Verification items for the finished model (mm, model axes). A direction names the side the tool comes from. Give positions to 0.01 mm unless a question says otherwise; leave off trailing zeros. Write each loop counter-clockwise with the first axis right and the second up, starting at its lowest first coordinate (ties: lowest second). Pieces come first, ordered by that corner, then holes.
Autodesk Inventor part; units mm, degrees
ref_plane "YZ Plane" through (0, 0, 0) normal (1, 0, 0) x (0, 1, 0)
ref_plane "XZ Plane" through (0, 0, 0) normal (0, 1, 0) x (-1, 0, 0)
ref_plane "XY Plane" through (0, 0, 0) normal (0, 0, 1) x (1, 0, 0)
sketch "Skizze1" plane through (0, 0, 0) normal (0, 0, 1) x (1, 0, 0)
  line L0 (-20.9977, -1.3) -> (5.0023, -1.3)
  line L1 (-22.2477, 0) -> (6.2523, 0)
  line L2 (-22.2477, 0) -> (-22.2477, -2.7)
  line L3 (-22.2477, -2.7) -> (-20.9977, -2.7)
  line L4 (-20.9977, -2.7) -> (-20.9977, -1.3)
  line L5 (5.0023, -1.3) -> (5.0023, -2.7)
  line L6 (5.0023, -2.7) -> (6.2523, -2.7)
  line L7 (6.2523, -2.7) -> (6.2523, 0)
  point P0 (0, 0)
  dimension "d0" = 26
  dimension "d1" = 28.5
  dimension "d2" = 1.25
  dimension "d33" = 1.3
  dimension "d37" = 2.7
  dimension "d38" = 2.7
  dimension "d39" = 0
extrude "Extrusion1" add sketch "Skizze1" along normal blind 25.5
sketch "Skizze2" plane through (0, 0, 0) normal (0, 0, -1) x (-1, 0, 0)
  line L0 (20.9977, -1.3) -> (-5.0023, -1.3)
  line L1 (20.9977, -2.7) -> (20.9977, -1.3)
  line L2 (-5.0023, -1.3) -> (-5.0023, -2.7)
  line L3 (0.9977, -1.3) -> (2.2477, -1.3)
  line L4 (2.2477, -1.3) -> (2.2477, -5.5195)
  line L5 (2.2477, -5.5195) -> (0.9977, -5.5195)
  line L6 (0.9977, -5.5195) -> (0.9977, -1.3)
  line L7 (13.7477, -1.3) -> (14.9977, -1.3)
  line L8 (14.9977, -1.3) -> (14.9977, -5.5195)
  line L9 (14.9977, -5.5195) -> (13.7477, -5.5195)
  line L10 (13.7477, -5.5195) -> (13.7477, -1.3)
  point P0 (0, 0)
  dimension "d5" = 11.5
  dimension "d6" = 1.25
  dimension "d7" = 1.25
  dimension "d8" = 6
  dimension "d9" = 6
extrude "Extrusion2" add sketch "Skizze2" against normal blind 16.35
sketch "Skizze3" plane through (0, 0, 0) normal (0, 0, -1) x (-1, 0, 0)
  line L0 (0.9977, -5.5195) -> (2.2477, -5.5195)
  line L1 (2.2477, -5.5195) -> (2.2477, -17.7695)
  line L2 (2.2477, -17.7695) -> (0.9977, -17.7695)
  line L3 (0.9977, -17.7695) -> (0.9977, -5.5195)
  line L4 (13.7477, -5.5195) -> (14.9977, -5.5195)
  line L5 (14.9977, -5.5195) -> (14.9977, -17.7695)
  line L6 (14.9977, -17.7695) -> (13.7477, -17.7695)
  line L7 (13.7477, -17.7695) -> (13.7477, -5.5195)
  point P0 (0, 0)
  dimension "d12" = 12.25
  dimension "d15" = 12.25
extrude "Extrusion3" add sketch "Skizze3" against normal blind 5
sketch "Skizze4" plane through (0, 0, 0) normal (0, 0, -1) x (-1, 0, 0)
  line L0 (0.9977, -17.7695) -> (2.2477, -17.7695)
  line L1 (2.2477, -17.7695) -> (2.2477, -24.0195)
  line L2 (2.2477, -24.0195) -> (0.9977, -24.0195)
  line L3 (0.9977, -24.0195) -> (0.9977, -17.7695)
  line L4 (13.7477, -17.7695) -> (14.9977, -17.7695)
  line L5 (14.9977, -17.7695) -> (14.9977, -24.0195)
  line L6 (14.9977, -24.0195) -> (13.7477, -24.0195)
  line L7 (13.7477, -24.0195) -> (13.7477, -17.7695)
  point P0 (0, 0)
  dimension "d16" = 6.25
  dimension "d17" = 6.25
extrude "Extrusion4" add sketch "Skizze4" against normal blind 16.35
sketch "Skizze5" plane through (-14.9977, -24.0195, 0) normal (0, -1, 0) x (1, 0, 0)
  line L0 (-7.25, 0) -> (-7.25, 25.5)
  line L1 (21.25, 0) -> (21.25, 25.5)
  line L2 (-7.25, 25.5) -> (-7.25, 0)
  line L3 (21.25, 0) -> (-7.25, 0)
  line L4 (21.25, 0) -> (21.25, 25.5)
  line L5 (21.25, 25.5) -> (18.8, 25.5)
  line L6 (18.8, 25.5) -> (18.8, 5.0223)
  line L7 (18.8, 5.0223) -> (15, 5.0223)
  line L8 (15, 5.0223) -> (15, 25.5)
  line L9 (15, 25.5) -> (6.75, 25.5)
  line L10 (6.75, 25.5) -> (6.75, 5.25)
  line L11 (6.75, 5.25) -> (-3.25, 5.25)
  line L12 (-3.25, 5.25) -> (-3.25, 25.5)
  line L13 (-3.25, 25.5) -> (-7.25, 25.5)
  point P0 (14.9977, 0)
  dimension "d20" = 5.25
  dimension "d21" = 8.25
  dimension "d22" = 3.8
  dimension "d23" = 10
  dimension "d24" = 4
  dimension "d25" = 2.45
extrude "Extrusion5" add sketch "Skizze5" against normal blind 1.3
sketch "Skizze6" plane through (-14.9977, -22.7195, 0) normal (0, 1, 0) x (1, 0, 0)
  line L0 (-3.25, -25.5) -> (-7.25, -25.5)
  line L1 (14, 0) -> (21.25, 0)
  line L2 (21.25, -25.5) -> (21.25, 0)
  line L3 (-7.25, 0) -> (-6, 0)
  line L4 (-6, 0) -> (-6, -25.5)
  line L5 (-6, -25.5) -> (-7.25, -25.5)
  line L6 (-7.25, -25.5) -> (-7.25, 0)
  line L7 (21.25, 0) -> (20, 0)
  line L8 (20, 0) -> (20, -25.5)
  line L9 (20, -25.5) -> (21.25, -25.5)
  line L10 (21.25, -25.5) -> (21.25, 0)
  point P0 (14.9977, 0)
  point P1 (18.8, -25.5)
  dimension "d28" = 1.25
  dimension "d30" = 1.25
extrude "Extrusion6" add sketch "Skizze6" along normal blind 1.3
sketch "Skizze7" plane through (0, 0, 0) normal (0, 0, -1) x (-1, 0, 0)
  line L0 (22.2477, 0) -> (22.2477, -2.7)
  line L1 (-6.2523, -2.7) -> (-6.2523, 0)
  line L2 (-13.1523, -8.7) -> (-10.1523, -8.7)
  line L3 (-10.1523, -8.7) -> (-10.1523, -10)
  line L4 (-10.1523, -10) -> (-13.1523, -10)
  line L5 (-13.1523, -10) -> (-13.1523, -8.7)
  line L6 (26.1477, -8.7) -> (29.1477, -8.7)
  line L7 (29.1477, -8.7) -> (29.1477, -10)
  line L8 (29.1477, -10) -> (26.1477, -10)
  line L9 (26.1477, -10) -> (26.1477, -8.7)
  line L10 (22.2477, -2.7) -> (20.9977, -2.7)
  line L11 (-5.0023, -2.7) -> (-6.2523, -2.7)
  point P0 (0, 0)
  dimension "d40" = 3.9
  dimension "d41" = 3.9
  dimension "d42" = 1.3
  dimension "d43" = 3
  dimension "d44" = 3
  dimension "d45" = 1.3
  dimension "d68" = 6
  dimension "d69" = 6
extrude "Extrusion7" add sketch "Skizze7" against normal blind 19.3
ref_plane "Arbeitsebene1" through (-22.2477, 3.5, 0) normal (0, 1, 0) x (1, 0, 0)
sketch "Skizze9" plane through (-22.2477, 3.5, 0) normal (0, 1, 0) x (1, 0, 0)
  line L0 (28.5, 0) -> (28.5, -25.5)
  line L1 (28.5, 0) -> (0, 0)
  line L2 (0, 0) -> (0, -25.5)
  line L3 (0.75, 0) -> (27.75, 0)
  line L4 (27.75, 0) -> (27.75, -19.8)
  line L5 (27.75, -19.8) -> (0.75, -19.8)
  line L6 (0.75, -19.8) -> (0.75, 0)
  point P0 (22.2477, 0)
  point P1 (22.2477, 0)
  dimension "d55" = 27
  dimension "d56" = 19.8
  dimension "d57" = 0.75
  dimension "d58" = 0.75
extrude "Extrusion9" add sketch "Skizze9" against normal blind 2
sketch "Skizze11" plane through (0, 0, 0) normal (0, 0, -1) x (-1, 0, 0)
  line L0 (22.2477, -24.0195) -> (22.2477, -21.4195)
  line L1 (22.2477, 0) -> (22.2477, -2.7)
  line L2 (-6.2523, -2.7) -> (-6.2523, 0)
  line L3 (-6.2523, -24.0195) -> (-6.2523, -21.4195)
  line L4 (-11.7523, -2.7) -> (-14.5023, -24.0195)
  line L5 (27.7477, -2.7) -> (30.4977, -24.0195)
  line L6 (-5.5023, 3.5) -> (-5.5023, 1.5)
  line L7 (21.4977, 3.5) -> (21.4977, 1.5)
  line L8 (-11.7523, -2.7) -> (-5.5023, 1.5)
  line L9 (-5.5023, 1.5) -> (-5.5023, 3.5)
  line L10 (27.7477, -2.7) -> (21.4977, 1.5)
  line L11 (21.4977, 1.5) -> (21.4977, 3.5)
  line L12 (21.4977, 3.5) -> (29.1227, -1.624)
  line L13 (29.1227, -1.624) -> (31.9868, -23.8275)
  line L14 (31.9868, -23.8275) -> (30.4977, -24.0195)
  line L15 (-5.5023, 1.5) -> (-5.5023, 3.5)
  line L16 (-5.5023, 3.5) -> (-13.1273, -1.624)
  line L17 (-13.1273, -1.624) -> (-15.9913, -23.8275)
  line L18 (-15.9913, -23.8275) -> (-14.5023, -24.0195)
  point P0 (0, 0)
  dimension "d65" = 28.5
  dimension "d66" = 8.25
  dimension "d67" = 8.25
  dimension "d70" = 5.5
  dimension "d71" = 5.5
extrude "Extrusion10" add sketch "Skizze11" against normal blind 18.7
sketch "Skizze12" plane through (0, 0, 0) normal (0, 0, -1) x (-1, 0, 0)
  line L0 (31.9868, -23.8275) -> (29.1227, -1.624)
  line L1 (29.1227, -1.624) -> (21.4977, 3.5)
  line L2 (21.4977, 3.5) -> (-5.5023, 3.5)
  line L3 (-5.5023, 3.5) -> (-13.1273, -1.624)
  line L4 (-13.1273, -1.624) -> (-15.9913, -23.8275)
  line L5 (-15.9913, -23.8275) -> (31.9868, -23.8275)
  point P0 (0, 0)
extrude "Extrusion11" add sketch "Skizze12" along normal blind 2
equation "\"d38\" = d37"
equation "\"d7\" = d6"
equation "\"d15\" = d12"
equation "\"d17\" = d16"
equation "\"d41\" = d40"
equation "\"d44\" = d43"
equation "\"d45\" = d42"
equation "\"d69\" = d68"
equation "\"d57\" = d58"
equation "\"d66\" = d67"
equation "\"d70\" = d71"
properties part number "conrad_schaltsteckdose"
Item 1: Depth check by flat-ended pin: pin 1 (1.4 mm diameter, centred on y = -23.5, z = 11.5, fed in from -X); pin 2 (1 mm diameter, centred on x = -11.5, y = -23, fed in from +Z); pin 3 (8 mm diameter, centred on y = -11.5, z = 1, fed in from -X); pin 4 (3.5 mm diameter, centred on x = 11.5, z = 12.5, fed in from +Y). Enter the tip coordinate at first touch or a pass-through.
Answer key:
pin 1: stops at x = -31.99
pin 2: stops at z = 5.25
pin 3: stops at x = -30.91
pin 4: stops at y = 0.65
Item 2: Sectioned sample at A-A on z = 20.5. Record the cut outline in (x, y), then the cut area to 3 significant figures.
Answer key:
outline: (-22.25, -24.02) - (-18.25, -24.02) - (-18.25, -22.72) - (-21, -22.72) - (-21, -21.42) - (-22.25, -21.42) - close; (-22.25, -2.7) - (-21, -2.7) - (-21, -1.3) - (5, -1.3) - (5, -2.7) - (6.25, -2.7) - (6.25, 0) - (-22.25, 0) - close; (-8.25, -24.02) - (0, -24.02) - (0, -22.72) - (-8.25, -22.72) - close; (3.8, -24.02) - (6.25, -24.02) - (6.25, -21.42) - (5, -21.42) - (5, -22.72) - (3.8, -22.72) - close
area: 62.9 mm2
Item 3: Sectioned sample at C-C on z = 2. State how many separate pieces and enclosed holes the cut face has, then the cut area to 3 significant figures.
Answer key:
separate pieces: 2
enclosed holes: 1
area: 288 mm2
Item 4: Scan lines: line 1 along Y through (x, z) = (-7.5, 15); line 2 along X through (y, z) = (-20.5, 6.5); line 3 along X through (y, z) = (-13, 1.5). Record each from-to range of solid material in increasing order.
Answer key:
line 1: y = -24.02 to -22.72, -1.3 to 0, 1.5 to 3.5
line 2: x = -31.56 to -30.04, -15 to -13.75, -2.25 to -1, 14.05 to 15.56
line 3: x = -30.59 to -29.08, -15 to -13.75, -2.25 to -1, 13.08 to 14.59
Item 5: Sectioned sample at D-D on y = -20.75. Record the cut outline in (x, z).
Answer key:
outline: (-31.59, -2) - (15.59, -2) - (15.59, 18.7) - (14.08, 18.7) - (14.08, 0) - (-1, 0) - (-1, 16.35) - (-2.25, 16.35) - (-2.25, 0) - (-13.75, 0) - (-13.75, 16.35) - (-15, 16.35) - (-15, 0) - (-30.08, 0) - (-30.08, 18.7) - (-31.59, 18.7) - close
Item 6: Release check for a two-part mould opening along Y. For faces 1 (the face through (5.002, -2, 13)), 2 (the face through (-8, -10, -2)), 3 (the face through (-30.575, -12.881, 8.495)) record: released by +Y, released by -Y, zero draft, split by the parting line, or undercut.
Answer key:
face 1: undercut
face 2: zero draft
face 3: released by +Y
Item 7: Sectioned sample at B-B on x = -1.5. Record the cut outline in (y, z).
Answer key:
outline: (-24.02, 0) - (-23.83, 0) - (-23.83, -2) - (3.5, -2) - (3.5, 19.8) - (1.5, 19.8) - (1.5, 0) - (0, 0) - (0, 25.5) - (-1.3, 25.5) - (-1.3, 16.35) - (-5.52, 16.35) - (-5.52, 5) - (-17.77, 5) - (-17.77, 16.35) - (-22.72, 16.35) - (-22.72, 25.5) - (-24.02, 25.5) - close
Item 8: Set-up check for faces 4 (the face through (12, -9, 19.3)), 5 (the face through (-22, -2.7, 13)), 6 (the face through (-17, -23, 5.25)): record each of +Z, -Z, +X, -X, +Y, -Y from which the full face is reachable in a straight line by a thin tool's end or side.
Answer key:
face 4: +Z, +X, -X, +Y, -Y
face 5: +Z
face 6: +Z, -Y
